Input: part model. Units: mm. Frame: model coordinates. A direction names the side the tool comes from. Round coordinates to 2 decimals unless told otherwise and drop trailing zeros. Loops run counter-clockwise (first coordinate to the right, second up) from the corner with the lowest first, then second, coordinate; pieces in that order, holes last. Notation, with made-up numbers: (28.25, 27) -> (61.25, 27) arc R18 ccw to (61.25, 58) -> close; hole circle Ø7 at (57.5, 65.25). An arc over 180 degrees is marked (long way). One line per question, with ' | ' between items. Start each with the question number.
Q1. Contact query for flat-ended pins moving along their axis: P1, Ø15, axis at x = 0, z = -55, coming from the -Y side; P2, Ø7.5, axis at x = 0, z = 55, coming from the -Y side; P3, Ø5, axis at y = -3.5, z = 17.5, coming from the +X side; P4, Ø7, axis at x = -24.5, z = 32, coming from the -Y side. Output: stop coordinate, or through.
Q2. Material intervals for L1, parallel to Z at x = 0, y = 0.75; L2, parallel to X at y = 6.5, z = 55; L3, parallel to X at y = -7, z = 55, sorted ascending.
Q3. Cut plane A-A on z = -55. Return loops of the section in (x, y).
Q4. Cut plane C-C on y = -7.75. Return loops of the section in (x, z).
Q5. Access query for faces 1 (the face through (-1.277, -2.605, 59.054)), 2 (the face through (26, 0, -1)), 3 (the face through (-27, 0, -1)), 4 (the face through (-1, 10, -1)), 5 (the face through (-1.95, 7.46, 61.2)). Directions: +Z, -Z, +X, -X, +Y, -Y. A direction counts if a zero-diameter tool reaches every point of the face in a straight line with its end or side. Return the directions, or none.
Q6. Mould query, pull axis X, two halves, no side actions, for faces 6 (the face through (-1.277, -2.605, -50.946)), 7 (the face through (4.2, 5, -53.6)), 8 (the face through (0, -10, -1)), 9 (the face through (-40, 5, 0)). Classes: pulls with the +X half, pulls with the -X half, needs draft (parallel to the pull), parting line crosses it, or undercut.
Q7. Cut plane B-B on x = 0. Return loops of the section in (y, z).
Q8. Cut plane D-D on z = 35.5. Return loops of the section in (x, y).
Autodesk Inventor part; units mm, degrees
ref_plane "YZ Plane" through (0, 0, 0) normal (1, 0, 0) x (0, 1, 0)
ref_plane "XZ Plane" through (0, 0, 0) normal (0, 1, 0) x (-1, 0, 0)
ref_plane "XY Plane" through (0, 0, 0) normal (0, 0, 1) x (1, 0, 0)
sketch "Sketch3" plane through (0, 0, 0) normal (0, 0, 1) x (1, 0, 0)
  line L0 (-40, 0) -> (-40, 10)
  line L1 (-40, 10) -> (40, 10)
  line L2 (40, 10) -> (40, 0)
  line L3 (-40, 0) -> (-15, 0)
  line L4 (-15, 0) -> (-15, -10)
  line L5 (-15, -10) -> (15, -10)
  line L6 (15, -10) -> (15, 0)
  line L7 (15, 0) -> (40, 0)
  point P0 (0, 0)
  dimension "d0" = 40
  dimension "d1" = 10
  dimension "d2" = 80
  dimension "d6" = 25
  dimension "d7" = 10
  dimension "d8" = 30
  dimension "d9" = 10
extrude "Extrusion1" add sketch "Sketch3" along normal mid plane 150
sketch "Sketch4" plane through (-40, 10, 75) normal (0, 1, 0) x (1, 0, 0)
  point P0 (40, 75)
chamfer "Chamfer1" distance 2 angle 45 15 edges at (0, 10, 75) (0, 10, -75) (15, -5, 75) (27.5, 0, 75) (40, 0, 0) (27.5, 0, -75) (40, 5, 75) (40, 10, 0) (40, 5, -75) (-15, -5, 75) (-27.5, 0, -75) (-40, 10, 0) (-40, 5, -75) (-40, 0, 0) (-27.5, 0, 75)
sketch "Sketch5" plane through (-38, 10, -73) normal (0, 1, 0) x (1, 0, 0)
  circle A0 centre (38, -18) radius 5.6308
  circle A1 centre (38, -128) radius 5.6351
  line L0 (-2, -148) -> (76, -148)
  line L1 (76, 2) -> (0, 2)
  line L2 (76, 0) -> (76, -146)
  line L3 (78, -146) -> (78, 0)
  point P0 (38, -73)
  dimension "d13" = 20
  dimension "d14" = 20
  dimension "d16" = 40
  dimension "d17" = 40
hole "Hole1" at (0, 10, -55) at (0, 10, 55) direction (0, -1, 0) diameter 8.5 end through all counterbore diameter 13 counterbore depth 5
properties part number "Hanging bracket male"
Results:
1) P1: y = -10 | P2: through | P3: x = 15 | P4: y = 0
2) L1: -75 to -59.25, -50.75 to 50.75, 59.25 to 75 | L2: -40 to -6.5, 6.5 to 40 | L3: -15 to -4.25, 4.25 to 15
3) outline: (-40, 2) -> (-38, 0) -> (-15, 0) -> (-15, -10) -> (-4.25, -10) -> (-4.25, 5) -> (-6.5, 5) -> (-6.5, 10) -> (-38, 10) -> (-40, 8) -> close; (4.25, -10) -> (15, -10) -> (15, 0) -> (38, 0) -> (40, 2) -> (40, 8) -> (38, 10) -> (6.5, 10) -> (6.5, 5) -> (4.25, 5) -> close
4) outline: (-15, -75) -> (15, -75) -> (15, 73) -> (13, 75) -> (-13, 75) -> (-15, 73) -> close; hole circle Ø8.5 at (0, -55); hole circle Ø8.5 at (0, 55)
5) face 1: +Y, -Y | face 2: +Z, -Z, +X, -Y | face 3: +Z, -Z, -X, -Y | face 4: +Z, -Z, +X, -X, +Y | face 5: +Y
6) face 6: undercut | face 7: undercut | face 8: needs draft | face 9: pulls with the -X half
7) outline: (-10, -75) -> (8, -75) -> (10, -73) -> (10, -61.5) -> (5, -61.5) -> (5, -59.25) -> (-10, -59.25) -> close; (-10, -50.75) -> (5, -50.75) -> (5, -48.5) -> (10, -48.5) -> (10, 48.5) -> (5, 48.5) -> (5, 50.75) -> (-10, 50.75) -> close; (-10, 59.25) -> (5, 59.25) -> (5, 61.5) -> (10, 61.5) -> (10, 73) -> (8, 75) -> (-10, 75) -> close
8) outline: (-40, 2) -> (-38, 0) -> (-15, 0) -> (-15, -10) -> (15, -10) -> (15, 0) -> (38, 0) -> (40, 2) -> (40, 8) -> (38, 10) -> (-38, 10) -> (-40, 8) -> close
